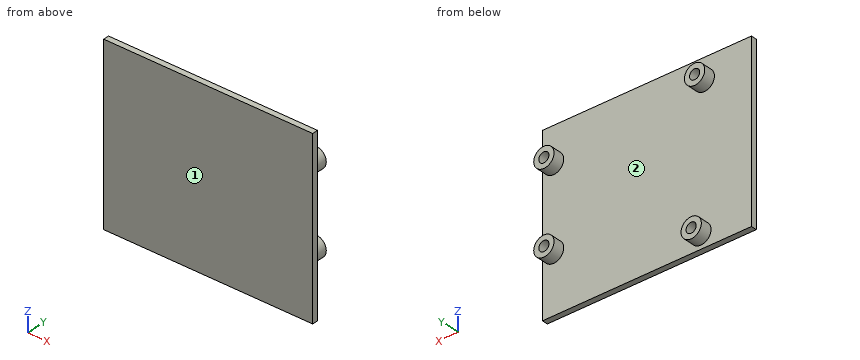
```python
from build123d import *

# Parameters (mm, degrees)
ESQUISSE1_W             = 72
ESQUISSE1_H             = 60
BOSS_EXTRU_1_DEPTH      = 2
ESQUISSE3_R             = 3.5
BOSS_EXTRU_2_DEPTH      = 4
ESQUISSE2_R             = 1.75
ENL_V_MAT_EXTRU_1_DEPTH = 4


with BuildPart() as part:
    # Esquisse1 → Boss.-Extru.1 (new body)
    with BuildSketch(Plane(origin=(0, 0, 0), x_dir=(1, 0, 0), z_dir=(0, 1, 0))):
        Rectangle(ESQUISSE1_W, ESQUISSE1_H)
    extrude(amount=BOSS_EXTRU_1_DEPTH)

    # Esquisse3 → Boss.-Extru.2 (add)
    with BuildSketch(Plane(origin=(0, 2, 0), x_dir=(1, 0, 0), z_dir=(0, 1, 0))):
        with Locations((-19.741989578, -22.677254534)):
            Circle(ESQUISSE3_R)
        with Locations((32.17700457, -17.941217791)):
            Circle(ESQUISSE3_R)
        with Locations((32.180787909, 9.986620664)):
            Circle(ESQUISSE3_R)
        with Locations((-18.564843267, 25.173313711)):
            Circle(ESQUISSE3_R)
    extrude(amount=BOSS_EXTRU_2_DEPTH)

    # Esquisse2 → Enlèv. mat.-Extru.1 (cut)
    with BuildSketch(Plane(origin=(0, 2, 0), x_dir=(1, 0, 0), z_dir=(0, 1, 0))):
        with Locations((-18.564843267, 25.173313711)):
            Circle(ESQUISSE2_R)
        with Locations((32.180787909, 9.986620664)):
            Circle(ESQUISSE2_R)
        with Locations((32.17700457, -17.941217791)):
            Circle(ESQUISSE2_R)
        with Locations((-19.741989578, -22.677254534)):
            Circle(ESQUISSE2_R)
    extrude(amount=ENL_V_MAT_EXTRU_1_DEPTH, mode=Mode.SUBTRACT)


solid = part.part
```
Model file for the job. Use its own axes, mm. Face numbers are marked on the shaded views. A direction names the side the tool comes from. Give positions to 0.01 mm unless a question says otherwise; leave off trailing zeros. Write each loop counter-clockwise with the first axis right and the second up, starting at its lowest first coordinate (ties: lowest second). Pieces come first, ordered by that corner, then holes. Notation, with made-up numbers: (58, 18.25) - (98, 18.25) arc R12 ccw to (98, 41.25) - close; hole circle Ø5 at (82.25, 47.25). An arc over 180 degrees is marked (long way). One line per question, with ' | ' between items. Start each with the question number.
(1) Slice it at A-A on y = 3.1. Write the cut outline in (x, z).
(2) Slice it at B-B on z = 1. Write the cut outline in (x, y), plus the area to 3 significant figures.
(3) Wall check: line 1 along Y through (x, z) = (-5, -18.5); line 2 along X through (y, z) = (5.6, -26); line 3 along X through (y, z) = (3.55, 20). Give the ranges that are in metal, low to high. Write a range as from..to.
(4) 3-axis set-ups, long thin cutter, end or side, ignore diameter. For the marked faces 1 and 2: which of +Z, -Z, +X, -X, +Y, -Y reach the whole face in a straight line?
(5) Slice it at C-C on x = 3.5. Write the cut outline in (y, z), plus the area to 3 significant figures.
(6) Pin check, flat tips, straight feed: P1, Ø6, axis at x = -7.5, z = -14.5, coming from the -Y side; P2, Ø2, axis at x = 32.18, z = -9.99, coming from the +Y side. Stop position of each tip, or through.
Results below:
1) outline: circle Ø7 at (-19.74, 22.68); circle Ø7 at (-18.56, -25.17); circle Ø7 at (32.18, -9.99); circle Ø7 at (32.18, 17.94); hole circle Ø3.5 at (-19.74, 22.68); hole circle Ø3.5 at (-18.56, -25.17); hole circle Ø3.5 at (32.18, -9.99); hole circle Ø3.5 at (32.18, 17.94)
2) outline: (-36, 0) - (36, 0) - (36, 2) - (-36, 2) - close | area: 144 mm^2
3) line 1: 0..2 | line 2: -21.97..-20.11, -17.02..-15.16 | line 3: -22..-17.49, 29.35..35.01
4) face 1: +Z, -Z, +X, -X, -Y | face 2: +Y
5) outline: (0, -30) - (2, -30) - (2, 30) - (0, 30) - close | area: 120 mm^2
6) P1: y = 0 | P2: y = 2
